The model under review builds one solid part; all positions refer to its coordinate system, in mm. A direction names the side the tool comes from. Round coordinates to 2 decimals unless told otherwise and drop trailing zeros. Order: outer loops, then holes, each group sorted by start corner. A loop starts at its lowest first (then second) coordinate and runs counter-clockwise, first axis right, second up. Notation, with made-up numbers: M -39.75,-12 L -30.75,-12 A24 ccw -30.75,2 Z; hole C -30,86.25 d10. An arc over 180 degrees is marked long. Answer as CSV lines item,"result". Start each with the question number.
from build123d import *

# Parameters (mm, degrees)
BOSS_EXTRUDE1_DEPTH = 38.1
SKETCH2_R           = 2.54
BOSS_EXTRUDE2_DEPTH = 6.35
LPATTERN1_COUNT     = 5
LPATTERN1_PITCH     = 52.3875
BOSS_EXTRUDE3_DEPTH = 25.4
CUT_EXTRUDE1_DEPTH  = 12.7


with BuildPart() as part:
    # Sketch1 → Boss-Extrude1 (new body)
    with BuildSketch(Plane(origin=(0, 0, 0), x_dir=(1, 0, 0), z_dir=(0, 1, 0))):
        Polygon((-69.85, 261.9375), (-69.85, 175.626209458), (-44.45, 169.276209458), (-44.45, 84.723790542), (-69.85, 78.373790542), (-69.85, -7.9375), (0, -25.4), (215.9, -25.4), (285.75, -7.9375), (285.75, 78.373790542), (260.35, 84.723790542), (260.35, 169.276209458), (285.75, 175.626209458), (285.75, 261.9375), (215.9, 279.4), (0, 279.4), align=None)
        Polygon((-25.4, 69.85), (-25.4, 184.15), (-50.8, 190.5), (-50.8, 241.3), (0, 254), (215.9, 254), (266.7, 241.3), (266.7, 190.5), (241.3, 184.15), (241.3, 69.85), (266.7, 63.5), (266.7, 12.7), (215.9, 0), (0, 0), (-50.8, 12.7), (-50.8, 63.5), align=None, mode=Mode.SUBTRACT)
    extrude(amount=BOSS_EXTRUDE1_DEPTH)

    # Sketch2 → Boss-Extrude2 (add)
    with BuildSketch(Plane(origin=(0, 0, 0), x_dir=(0, 0, -1), z_dir=(1, 0, 0))):
        with BuildLine():
            Line((-40.036226007, 23.553987204), (-25.4, 38.1))
            Line((-25.4, 38.1), (-25.4, 0))
            Line((-25.4, 0), (-40.036226007, 14.546012796))
            ThreePointArc((-40.036226007, 14.546012796), (-41.91, 19.05), (-40.036226007, 23.553987204))
        make_face()
        with Locations((-35.56, 19.05)):
            Circle(SKETCH2_R, mode=Mode.SUBTRACT)
    boss_extrude2 = extrude(amount=BOSS_EXTRUDE2_DEPTH)

    # LPattern1: Boss-Extrude2 ×5
    with Locations(*[(i * LPATTERN1_PITCH, 0, 0) for i in range(1, LPATTERN1_COUNT)]):
        add(boss_extrude2)

    # Sketch1<3> → Boss-Extrude3 (add)
    with BuildSketch(Plane(origin=(0, 0, 0), x_dir=(1, 0, 0), z_dir=(0, 1, 0))):
        Polygon((0, 76.2), (0, 177.8), (-25.4, 184.15), (-25.4, 69.85), align=None)
        Polygon((241.3, 69.85), (241.3, 184.15), (215.9, 177.8), (215.9, 76.2), align=None)
    extrude(amount=BOSS_EXTRUDE3_DEPTH)

    # Sketch1<4> → Cut-Extrude1 (cut)
    with BuildSketch(Plane(origin=(0, 0, 0), x_dir=(1, 0, 0), z_dir=(0, 1, 0))):
        Polygon((0, 76.2), (0, 177.8), (-25.4, 184.15), (-25.4, 69.85), align=None)
        Polygon((241.3, 69.85), (241.3, 184.15), (215.9, 177.8), (215.9, 76.2), align=None)
    extrude(amount=CUT_EXTRUDE1_DEPTH, mode=Mode.SUBTRACT)


solid = part.part
Item 1: The part is to be moulded in two halves that separate along Z. For faces 5 (the flat face through (285.75, 19, -35)), 6 (the flat face through (55.518, 7.171, 32.616)), 7 (the flat face through (-30.689, 18.783, -185.472)), 8 (the flat face through (109, 19, -279.4)), say which applies: +Z half, -Z half, draft (parallel to the pull), parting line (faces both ways), or undercut.
Item 2: For pin 1 (2 mm diameter, centred on x = 161, y = 28.5, fed in from +Z); pin 2 (6 mm diameter, centred on y = 12, z = -123, fed in from +X); pin 3 (12.5 mm diameter, centred on x = 222.5, z = -113.5, fed in from -Y), all flat-tipped, find the tip position at first contact; note any pin that passes through.
Item 3: Tool access review of faces 1 (the flat face through (-13, 12.7, -128)), 2 (the flat face through (-50.8, 19, -38)), 3 (the flat face through (-56.972, 18.783, -81.593)), 4 (the flat face through (134, 19, 25.4)): name each direction out of +Z, -Z, +X, -X, +Y, -Y from which nothing blocks a thin tool from reaching the whole face with its end or side.
Item 4: Consider section B-B (z = -55.5). State the section outline as (x, y) points, and give its area (3 significant figures).
Item 5: Wall thickness on probe 1 along Z at (x, y) = (3, 19); probe 2 along X at (y, z) = (31.5, -49); probe 3 along X at (y, z) = (37, -77.5): over which ranges is each line inside the solid? List them lowest first. Write a range as [from, to].
Item 6: Consider section A-A (x = 22.5). State the section outline as (y, z) points, and give its area (3 significant figures).
Reported:
1,face 5,"draft"
1,face 6,"+Z half"
1,face 7,"undercut"
1,face 8,"-Z half"
2,pin 1,"stops at z = 36.07"
2,pin 2,"stops at x = 260.35"
2,pin 3,"stops at y = 12.7"
3,face 1,"-Y"
3,face 2,"+Y, -Y"
3,face 3,"-X, +Y, -Y"
3,face 4,"+Z, +Y, -Y"
4,outline,"M -69.85,0 L -50.8,0 L -50.8,38.1 L -69.85,38.1 Z; M 266.7,0 L 285.75,0 L 285.75,38.1 L 266.7,38.1 Z"
4,area,"1,450 mm²"
5,probe 1,"z = [-279.4, -254], [0, 33.02], [38.1, 41.91]"
5,probe 2,"x = [-69.85, -50.8], [266.7, 285.75]"
5,probe 3,"x = [-69.85, -25.4], [241.3, 285.75]"
6,outline,"M 0,-279.4 L 38.1,-279.4 L 38.1,-254 L 0,-254 Z; M 0,0 L 38.1,0 L 38.1,25.4 L 0,25.4 Z"
6,area,"1,940 mm²"
